For this review, take the finished solid that the model builds, in its own axes (mm). Face numbers are marked on the shaded views. A direction names the side the tool comes from. Coordinates: 2 decimals unless noted, no trailing zeros. Order: outer loops, then holes, each group sorted by start corner. A loop starts at its lowest first (then second) coordinate and runs counter-clockwise, first axis right, second up. Notation, with made-up numbers: (63.5, -9.5) -> (110.5, -9.5) arc R21 ccw to (110.5, 25.5) -> close; hole circle Ø7 at (51, -32). An arc over 180 degrees is marked (long way). Answer as a JSON object with one key per item and string values. Group by question number.
1) Add section D-D, the plane z = 11.5. Count the separate pieces of the cut face and the enclosed holes in it, then the cut area to 4 significant figures.
2) Add section C-C, the plane x = 0. Write out the cut boundary in (y, z), then the cut area to 3 significant figures.
3) Draft analysis for pull direction X (two halves, no side actions). For the marked faces 1, 2, 3 and 4, state which applies: +X half, -X half, draft (parallel to the pull), parting line (faces both ways), or undercut.
4) Wall thickness on L1, parallel to X at y = 8, z = 3.5; L2, parallel to Y at x = 6.5, z = -4; L3, parallel to Y at x = -8.5, z = 8: over which ranges is each line inside the solid? List them lowest first.
5) Add section B-B, the plane z = 3. Write out the cut boundary in (x, y), then the cut area to 4 significant figures.
6) Machinability: for the marked faces 5, 6 and 7, which of the approach directions +Z, -Z, +X, -X, +Y, -Y give a long, thin tool a straight path to every point of the face, cutting with its end or side? Answer none if there is none.
7) Add section A-A, the plane y = 3.25. Write out the cut boundary in (x, z).
8) For pin 1 (1.1 mm diameter, centred on x = -9, z = -1, fed in from +Y); pin 2 (1.2 mm diameter, centred on y = 9.5, z = 3, fed in from +X); pin 3 (0.8 mm diameter, centred on y = 8, z = -1.5, fed in from -X); pin 4 (5 mm diameter, centred on x = -3, z = -3, fed in from +Y), all flat-tipped, find the tip position at first contact; note any pin that passes through.
from build123d import *

# Parameters (mm, degrees)
BASE_EXTRUDE_DEPTH        = 0.75
SIDEWALL_EXTRUDE_DEPTH    = 5.75
TOP_EXTRUDE_START         = 5.75
TOP_EXTRUDE_DEPTH         = 0.75
CUT_EXTRUDE1_DEPTH        = 29.901773302
CUT_EXTRUDE1_DEPTH_BACK   = 29.901773302
PCB_SUPPORT_EXTRUDE_DEPTH = 1
PCB_RIM_EXTRUDE_DEPTH     = 3.5
CUT_EXTRUDE2_DEPTH        = 21.941883869
CUT_EXTRUDE3_DEPTH        = 3.5


with BuildPart() as part:
    # battery-base → base-extrude (new body)
    with BuildSketch(Plane(origin=(0, 0, 0), x_dir=(1, 0, 0), z_dir=(0, 1, 0))):
        with BuildLine():
            Line((-10.5, 16.25), (10.5, 16.25))
            ThreePointArc((10.5, 16.25), (11.207106781, 15.957106781), (11.5, 15.25))
            Line((11.5, 15.25), (11.5, -13.75))
            ThreePointArc((11.5, -13.75), (11.207106781, -14.457106781), (10.5, -14.75))
            Line((10.5, -14.75), (-10.5, -14.75))
            ThreePointArc((-10.5, -14.75), (-11.207106781, -14.457106781), (-11.5, -13.75))
            Line((-11.5, -13.75), (-11.5, 15.25))
            ThreePointArc((-11.5, 15.25), (-11.207106781, 15.957106781), (-10.5, 16.25))
        make_face()
    extrude(amount=BASE_EXTRUDE_DEPTH)

    # battery-base_12 → sidewall-extrude (add)
    with BuildSketch(Plane(origin=(0, 0, 0), x_dir=(1, 0, 0), z_dir=(0, 1, 0))):
        with BuildLine():
            Line((-11.5, -13.5), (-10.75, -13.5))
            Line((-10.75, -13.5), (-10.75, 15))
            ThreePointArc((-10.75, 15), (-10.603553391, 15.353553391), (-10.25, 15.5))
            Line((-10.25, 15.5), (10.25, 15.5))
            ThreePointArc((10.25, 15.5), (10.603553391, 15.353553391), (10.75, 15))
            Line((10.75, 15), (10.75, -13.5))
            Line((10.75, -13.5), (11.5, -13.5))
            Line((11.5, -13.5), (11.5, 15.25))
            ThreePointArc((11.5, 15.25), (11.207106781, 15.957106781), (10.5, 16.25))
            Line((10.5, 16.25), (-10.5, 16.25))
            ThreePointArc((-10.5, 16.25), (-11.207106781, 15.957106781), (-11.5, 15.25))
            Line((-11.5, 15.25), (-11.5, -13.5))
        make_face()
    extrude(amount=SIDEWALL_EXTRUDE_DEPTH)

    # battery-base_13 → top-extrude (add)
    with BuildSketch(Plane(origin=(0, 0, 0), x_dir=(1, 0, 0), z_dir=(0, 1, 0)).offset(TOP_EXTRUDE_START)):
        with BuildLine():
            Line((10.75, 15), (10.75, -13.5))
            ThreePointArc((10.75, -13.5), (10.603553391, -13.853553391), (10.25, -14))
            Line((10.25, -14), (-10.25, -14))
            ThreePointArc((-10.25, -14), (-10.603553391, -13.853553391), (-10.75, -13.5))
            Line((-10.75, -13.5), (-10.75, 15))
            ThreePointArc((-10.75, 15), (-10.603553391, 15.353553391), (-10.25, 15.5))
            Line((-10.25, 15.5), (10.25, 15.5))
            ThreePointArc((10.25, 15.5), (10.603553391, 15.353553391), (10.75, 15))
        make_face()
        with BuildLine():
            ThreePointArc((-10.25, -14), (-10.603553391, -13.853553391), (-10.75, -13.5))
            Line((-10.75, -13.5), (-11.5, -13.5))
            Line((-11.5, -13.5), (-11.5, -13.75))
            ThreePointArc((-11.5, -13.75), (-11.207106781, -14.457106781), (-10.5, -14.75))
            Line((-10.5, -14.75), (10.5, -14.75))
            ThreePointArc((10.5, -14.75), (11.207106781, -14.457106781), (11.5, -13.75))
            Line((11.5, -13.75), (11.5, -13.5))
            Line((11.5, -13.5), (10.75, -13.5))
            ThreePointArc((10.75, -13.5), (10.603553391, -13.853553391), (10.25, -14))
            Line((10.25, -14), (-10.25, -14))
        make_face()
        with BuildLine():
            Line((-11.5, -13.5), (-10.75, -13.5))
            Line((-10.75, -13.5), (-10.75, 15))
            ThreePointArc((-10.75, 15), (-10.603553391, 15.353553391), (-10.25, 15.5))
            Line((-10.25, 15.5), (10.25, 15.5))
            ThreePointArc((10.25, 15.5), (10.603553391, 15.353553391), (10.75, 15))
            Line((10.75, 15), (10.75, -13.5))
            Line((10.75, -13.5), (11.5, -13.5))
            Line((11.5, -13.5), (11.5, 15.25))
            ThreePointArc((11.5, 15.25), (11.207106781, 15.957106781), (10.5, 16.25))
            Line((10.5, 16.25), (-10.5, 16.25))
            ThreePointArc((-10.5, 16.25), (-11.207106781, 15.957106781), (-11.5, 15.25))
            Line((-11.5, 15.25), (-11.5, -13.5))
        make_face()
    extrude(amount=TOP_EXTRUDE_DEPTH)

    # round-cut → Cut-Extrude1 (cut, two sides: drawn at the far end of the back side and taken through both)
    with BuildSketch(Plane(origin=(11.5, 0, 0), x_dir=(0, 0, -1), z_dir=(1, 0, 0)).offset(-CUT_EXTRUDE1_DEPTH_BACK)):
        with BuildLine():
            Line((-84.101155105, 0.75), (-13.5, 0.75))
            ThreePointArc((-13.5, 0.75), (-11, 3.25), (-13.5, 5.75))
            Line((-13.5, 5.75), (-84.101155105, 5.75))
            Line((-84.101155105, 5.75), (-225.303465314, 5.75))
            Line((-225.303465314, 5.75), (-225.303465314, 0.75))
            Line((-225.303465314, 0.75), (-84.101155105, 0.75))
        make_face()
    extrude(amount=CUT_EXTRUDE1_DEPTH + CUT_EXTRUDE1_DEPTH_BACK, mode=Mode.SUBTRACT)

    # PCB-support → PCB-support-extrude (add)
    with BuildSketch(Plane(origin=(0, 6.5, 0), x_dir=(1, 0, 0), z_dir=(0, 1, 0))):
        with BuildLine():
            Line((-8.75, -14), (-8.25, -14))
            Line((-8.25, -14), (-8.25, 15.5))
            Line((-8.25, 15.5), (-8.75, 15.5))
            ThreePointArc((-8.75, 15.5), (-9.103553391, 15.353553391), (-9.25, 15))
            Line((-9.25, 15), (-9.25, -13.5))
            ThreePointArc((-9.25, -13.5), (-9.103553391, -13.853553391), (-8.75, -14))
        make_face()
        with BuildLine():
            Line((8.25, 15.5), (8.25, -14))
            Line((8.25, -14), (8.75, -14))
            ThreePointArc((8.75, -14), (9.103553391, -13.853553391), (9.25, -13.5))
            Line((9.25, -13.5), (9.25, 15))
            ThreePointArc((9.25, 15), (9.103553391, 15.353553391), (8.75, 15.5))
            Line((8.75, 15.5), (8.25, 15.5))
        make_face()
    extrude(amount=PCB_SUPPORT_EXTRUDE_DEPTH)

    # PCB-support_3 → PCB-rim-extrude (add)
    with BuildSketch(Plane(origin=(0, 6.5, 0), x_dir=(1, 0, 0), z_dir=(0, 1, 0))):
        with BuildLine():
            Line((-8.25, -14.75), (-8.25, -14))
            Line((-8.25, -14), (-8.75, -14))
            ThreePointArc((-8.75, -14), (-9.103553391, -13.853553391), (-9.25, -13.5))
            Line((-9.25, -13.5), (-9.25, 15))
            ThreePointArc((-9.25, 15), (-9.103553391, 15.353553391), (-8.75, 15.5))
            Line((-8.75, 15.5), (-8.25, 15.5))
            Line((-8.25, 15.5), (-8.25, 16.25))
            Line((-8.25, 16.25), (-9, 16.25))
            ThreePointArc((-9, 16.25), (-9.707106781, 15.957106781), (-10, 15.25))
            Line((-10, 15.25), (-10, -13.75))
            ThreePointArc((-10, -13.75), (-9.707106781, -14.457106781), (-9, -14.75))
            Line((-9, -14.75), (-8.25, -14.75))
        make_face()
        with BuildLine():
            Line((8.75, -14), (8.25, -14))
            Line((8.25, -14), (8.25, -14.75))
            Line((8.25, -14.75), (9, -14.75))
            ThreePointArc((9, -14.75), (9.707106781, -14.457106781), (10, -13.75))
            Line((10, -13.75), (10, 15.25))
            ThreePointArc((10, 15.25), (9.707106781, 15.957106781), (9, 16.25))
            Line((9, 16.25), (8.25, 16.25))
            Line((8.25, 16.25), (8.25, 15.5))
            Line((8.25, 15.5), (8.75, 15.5))
            ThreePointArc((8.75, 15.5), (9.103553391, 15.353553391), (9.25, 15))
            Line((9.25, 15), (9.25, -13.5))
            ThreePointArc((9.25, -13.5), (9.103553391, -13.853553391), (8.75, -14))
        make_face()
    extrude(amount=PCB_RIM_EXTRUDE_DEPTH)

    # cut-away → Cut-Extrude2 (cut, through all)
    with BuildSketch(Plane(origin=(0, 6.5, 0), x_dir=(1, 0, 0), z_dir=(0, 1, 0))):
        with BuildLine():
            Line((-5, 7.75), (-5, -14.75))
            Line((-5, -14.75), (5, -14.75))
            Line((5, -14.75), (5, 7.75))
            ThreePointArc((5, 7.75), (0, 12.75), (-5, 7.75))
        make_face()
    extrude(amount=-CUT_EXTRUDE2_DEPTH, mode=Mode.SUBTRACT)

    # Sketch7 → Cut-Extrude3 (cut)
    with BuildSketch(Plane(origin=(0, 0, -16.25), x_dir=(-1, 0, 0), z_dir=(0, 0, -1))):
        with BuildLine():
            Line((8.584888193, 1.75), (-8.584888193, 1.75))
            ThreePointArc((-8.584888193, 1.75), (-10.084888193, 3.25), (-8.584888193, 4.75))
            Line((-8.584888193, 4.75), (8.584888193, 4.75))
            ThreePointArc((8.584888193, 4.75), (10.084888193, 3.25), (8.584888193, 1.75))
        make_face()
    extrude(amount=-CUT_EXTRUDE3_DEPTH, mode=Mode.SUBTRACT)


solid = part.part
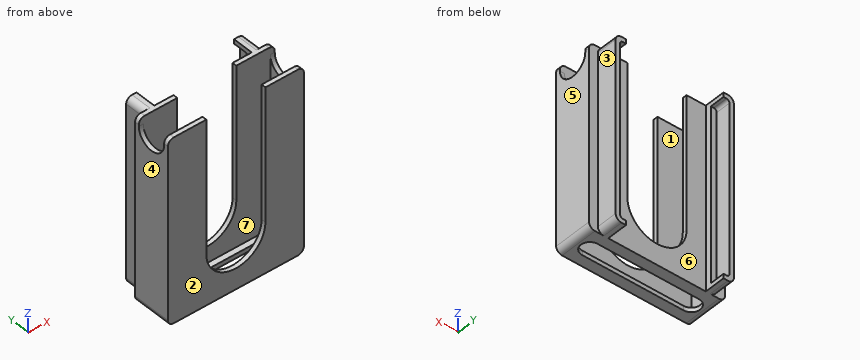
Output values:
{
 "1": {"separate pieces": "4", "enclosed holes": "0", "area": "29.75 mm²"},
 "2": {"outline": "(0, -16.25) -> (1.75, -16.25) -> (1.75, -15.5) -> (0.75, -15.5) -> (0.75, -12.75) -> (0, -12.75) -> close; (4.75, -16.25) -> (6.5, -16.25) -> (6.5, -12.75) -> (5.75, -12.75) -> (5.75, -15.5) -> (4.75, -15.5) -> close", "area": "6.75 mm²"},
 "3": {"face 1": "undercut", "face 2": "draft", "face 3": "+X half", "face 4": "-X half"},
 "4": {"L1": "x = -10 to -9.25, 9.25 to 10", "L2": "y = 0 to 0.75, 5.75 to 6.5", "L3": "y = 0 to 0.75, 5.75 to 7.5"},
 "5": {"outline": "(-11.5, 0) -> (-5, 0) -> (-5, 0.75) -> (-10.75, 0.75) -> (-10.75, 5.75) -> (-5, 5.75) -> (-5, 6.5) -> (-8.25, 6.5) -> (-8.25, 7.5) -> (-9.25, 7.5) -> (-9.25, 10) -> (-10, 10) -> (-10, 6.5) -> (-11.5, 6.5) -> close; (5, 0) -> (11.5, 0) -> (11.5, 6.5) -> (10, 6.5) -> (10, 10) -> (9.25, 10) -> (9.25, 7.5) -> (8.25, 7.5) -> (8.25, 6.5) -> (5, 6.5) -> (5, 5.75) -> (10.75, 5.75) -> (10.75, 0.75) -> (5, 0.75) -> close", "area": "34.25 mm²"},
 "6": {"face 5": "+Z, -Z, +X, +Y, -Y", "face 6": "+Z, -Z, +Y", "face 7": "+Z"},
 "7": {"outline": "(-11.5, -15.25) arc R1 ccw to (-10.5, -16.25) -> (-10.08, -16.25) -> (-10.08, -15.5) -> (-10.25, -15.5) arc R0.5 cw to (-10.75, -15) -> (-10.75, 11) -> (-11.5, 11) -> close; (10.08, -16.25) -> (10.5, -16.25) arc R1 ccw to (11.5, -15.25) -> (11.5, 11) -> (10.75, 11) -> (10.75, -15) arc R0.5 cw to (10.25, -15.5) -> (10.08, -15.5) -> close"},
 "8": {"pin 1": "stops at y = 10", "pin 2": "stops at x = 10", "pin 3": "stops at x = -10", "pin 4": "stops at y = 6.5"}
}
